Geometry check sheet. Reference: the model listing, model coordinates, mm. A direction names the side the tool comes from. Round coordinates to 2 decimals unless told otherwise and drop trailing zeros. Loops run counter-clockwise (first coordinate to the right, second up) from the corner with the lowest first, then second, coordinate; pieces in that order, holes last. Notation, with made-up numbers: (47, -29.75) -> (55, -29.75) arc R21 cw to (55, -20.75) -> close; hole circle Ø3 at (69.5, -36.5). An arc over 180 degrees is marked (long way). Use a Markdown table: item, result. Add a question column.
Q1. Release check for a two-part mould opening along Y. For faces 6 (the face through (1, 4, 15.593)), 7 (the face through (1, -8.874, -12)), 8 (the face through (1.48, -4.27, -3.59)) record: released by +Y, released by -Y, zero draft, split by the parting line, or undercut.
Q2. Material ranges on L1, parallel to Y at x = 2.35, z = -10; L2, parallel to Z at x = 1.95, y = -9.5; L3, parallel to Z at x = 1, y = -14.25, recorded low to high.
Q3. Sectioned sample at B-B, the plane z = -14. Enter the section's corners in (x, y).
Q4. Sectioned sample at D-D, the plane y = -4. Enter the section's corners in (x, z).
Q5. Set-up check for faces 1 (the face through (1, 2.126, -15)), 2 (the face through (1, -17.874, -15)), 3 (the face through (3, -8, 1)), 4 (the face through (1, 5.126, 13)), 5 (the face through (1, -0.374, -10)): record each of +Z, -Z, +X, -X, +Y, -Y from which the full face is reachable in a straight line by a thin tool's end or side.
Q6. Sectioned sample at A-A, the plane y = -17. Enter the section's corners in (x, z), then the cut area to 3 significant figures.
Q7. Sectioned sample at C-C, the plane z = -2. Enter the section's corners in (x, y).
Q8. Gauge pin test, flat ends, axial feed: P1, Ø1.5, axis at x = 2, z = -11.5, coming from the -Y side; P2, Ø0.5, axis at x = 2, z = 16.5, coming from the +Y side; P3, Ø1, axis at y = -7, z = 10, coming from the -X side; P4, Ø0.8, axis at x = 1, z = -14.5, coming from the -Y side. Record the tip position at first contact, or that the pin passes through.
```python
from build123d import *

# Parameters (mm, degrees)
RESSALTO_EXTRUS_O1_DEPTH = 3


with BuildPart() as part:
    # Esboço1 → Ressalto-extrusão1 (new body)
    with BuildSketch(Plane(origin=(0, 0, 0), x_dir=(0, 0, -1), z_dir=(1, 0, 0))):
        Polygon((-15.593145924, 2.125903998), (-17.093145924, 2.125903998), (-17.093145924, -17.874096002), (-15.593145924, -17.874096002), (-15.593145924, -20.874096002), (-10.593145924, -20.874096002), (-10.593145924, -17.874096002), (-9.093145924, -17.874096002), (10.406854076, -17.874096002), (10.406854076, -15.374096002), (9.031854076, -15.374096002), (9.031854076, -12.874096002), (10.406854076, -12.874096002), (10.406854076, -10.374096002), (10.406854076, -8.874096002), (13.406854076, -8.874096002), (13.406854076, -10.374096002), (13.406854076, -12.874096002), (14.781854076, -12.874096002), (14.781854076, -15.374096002), (13.406854076, -15.374096002), (13.406854076, -17.874096002), (15.906854076, -17.874096002), (15.906854076, 2.125903998), (13.406854076, 2.125903998), (13.406854076, -0.374096002), (14.781854076, -0.374096002), (14.781854076, -2.874096002), (13.406854076, -2.874096002), (13.406854076, -5.374096002), (13.406854076, -6.874096002), (10.406854076, -6.874096002), (10.406854076, -5.374096002), (10.406854076, -3.256067355), (10.406854076, -2.874096002), (9.031854076, -2.874096002), (9.031854076, -0.374096002), (10.406854076, -0.374096002), (10.406854076, 2.125903998), (-9.093145924, 2.125903998), (-10.593145924, 2.125903998), (-10.593145924, 5.125903998), (-15.593145924, 5.125903998), align=None)
        with BuildLine():
            Line((-7.953248379, -9.515906406), (-13.522081436, -13.389877228))
            ThreePointArc((-13.522081436, -13.389877228), (-14.556252559, -13.455274595), (-15.093145924, -12.568972026))
            Line((-15.093145924, -12.568972026), (-15.093145924, -3.179219979))
            ThreePointArc((-15.093145924, -3.179219979), (-14.556252559, -2.292917409), (-13.522081436, -2.358314777))
            Line((-13.522081436, -2.358314777), (-7.953248379, -6.232285599))
            ThreePointArc((-7.953248379, -6.232285599), (-7.095377355, -7.874096002), (-7.953248379, -9.515906406))
        make_face(mode=Mode.SUBTRACT)
        with BuildLine():
            Line((-4.7352749, -10.059924856), (-10.475594696, -14.053190801))
            ThreePointArc((-10.475594696, -14.053190801), (-10.858706607, -15.173340717), (-9.904530208, -15.874096002))
            Line((-9.904530208, -15.874096002), (2.71823836, -15.874096002))
            ThreePointArc((2.71823836, -15.874096002), (3.67241476, -15.173340717), (3.289302849, -14.053190801))
            Line((3.289302849, -14.053190801), (-2.451016947, -10.059924856))
            ThreePointArc((-2.451016947, -10.059924856), (-3.593145924, -9.701735259), (-4.7352749, -10.059924856))
        make_face(mode=Mode.SUBTRACT)
        with BuildLine():
            Line((0.766956531, -9.515906406), (6.335789588, -13.389877228))
            ThreePointArc((6.335789588, -13.389877228), (7.369960712, -13.455274595), (7.906854076, -12.568972026))
            Line((7.906854076, -12.568972026), (7.906854076, -10.374096002))
            Line((7.906854076, -10.374096002), (7.906854076, -3.179219979))
            ThreePointArc((7.906854076, -3.179219979), (7.369960712, -2.292917409), (6.335789588, -2.358314777))
            Line((6.335789588, -2.358314777), (0.766956531, -6.232285599))
            ThreePointArc((0.766956531, -6.232285599), (-0.090914492, -7.874096002), (0.766956531, -9.515906406))
        make_face(mode=Mode.SUBTRACT)
        with BuildLine():
            Line((3.289302849, -1.695001204), (-2.451016947, -5.688267149))
            ThreePointArc((-2.451016947, -5.688267149), (-3.593145924, -6.046456746), (-4.7352749, -5.688267149))
            Line((-4.7352749, -5.688267149), (-10.475594696, -1.695001204))
            ThreePointArc((-10.475594696, -1.695001204), (-10.858706607, -0.574851288), (-9.904530208, 0.125903998))
            Line((-9.904530208, 0.125903998), (2.71823836, 0.125903998))
            ThreePointArc((2.71823836, 0.125903998), (3.67241476, -0.574851288), (3.289302849, -1.695001204))
        make_face(mode=Mode.SUBTRACT)
    extrude(amount=RESSALTO_EXTRUS_O1_DEPTH)


solid = part.part
```
Values:
| question | item | result |
|---|---|---|
| 1 | face 6 | zero draft |
| 1 | face 7 | released by -Y |
| 1 | face 8 | undercut |
| 2 | L1 | -17.87 to -15.37, -12.87 to -2.87, -0.37 to 2.13 |
| 2 | L2 | -15.91 to -13.41, -10.41 to -7.91, -0.74 to 7.93, 15.09 to 17.09 |
| 2 | L3 | -15.91 to -14.78, -9.03 to -3.5, 10.69 to 17.09 |
| 3 | outline | (0, -17.87) -> (3, -17.87) -> (3, -15.37) -> (0, -15.37) -> close; (0, -12.87) -> (3, -12.87) -> (3, -2.87) -> (0, -2.87) -> close; (0, -0.37) -> (3, -0.37) -> (3, 2.13) -> (0, 2.13) -> close |
| 4 | outline | (0, -15.91) -> (3, -15.91) -> (3, -13.41) -> (0, -13.41) -> close; (0, -10.41) -> (3, -10.41) -> (3, -7.91) -> (0, -7.91) -> close; (0, -3.98) -> (3, -3.98) -> (3, 0.02) -> (0, 0.02) -> close; (0, 7.16) -> (3, 7.16) -> (3, 11.16) -> (0, 11.16) -> close; (0, 15.09) -> (3, 15.09) -> (3, 17.09) -> (0, 17.09) -> close |
| 5 | face 1 | -Z, +X, -X, +Y |
| 5 | face 2 | -Z, +X, -X, -Y |
| 5 | face 3 | +Z, -Z, +X, +Y, -Y |
| 5 | face 4 | +Z, -Z, +X, -X, +Y |
| 5 | face 5 | +X, -X |
| 6 | outline | (0, -15.91) -> (3, -15.91) -> (3, -13.41) -> (0, -13.41) -> close; (0, -10.41) -> (3, -10.41) -> (3, 17.09) -> (0, 17.09) -> close |
| 6 | area | 90.0 mm^2 |
| 7 | outline | (0, -17.87) -> (3, -17.87) -> (3, -15.87) -> (0, -15.87) -> close; (0, -13.16) -> (3, -13.16) -> (3, -10.37) -> (0, -10.37) -> close; (0, -5.37) -> (3, -5.37) -> (3, -2.59) -> (0, -2.59) -> close; (0, 0.13) -> (3, 0.13) -> (3, 2.13) -> (0, 2.13) -> close |
| 8 | P1 | y = -8.87 |
| 8 | P2 | y = 2.13 |
| 8 | P3 | through |
| 8 | P4 | y = -17.87 |
